For this review, take the finished solid that the model builds, in its own axes (mm). A direction names the side the tool comes from. Give positions to 0.01 mm unless a question says otherwise; leave off trailing zeros. Write each loop counter-clockwise with the first axis right and the second up, starting at its lowest first coordinate (ties: lowest second). Pieces come first, ordered by that corner, then holes. Notation, with made-up numbers: M 84.5,47.5 L 112.5,47.5 A25 ccw 112.5,82.5 Z; hole C 42.25,80 d10. An arc over 180 degrees is marked long. Use one line per item in the form item = value. Start each with the question number.
Q1. Consider section C-C on y = 25.5. Write out the cut boundary in (x, z), and give its area (3 significant figures).
Q2. Clearance check with flat-ended pins moving along their axes: pin 1 Ø24.5 at (x, y) = (-18.5, 43.5) entering from -Z; pin 2 Ø5 at (y, z) = (88.5, 21.5) entering from +X; pin 3 Ø6 at (x, z) = (102.5, -33.5) entering from +Y. State where each tip first meets the part, or that it passes through.
Q3. Tool access review of faces 1 (the flat face through (-2, 42, -90)), 2 (the cylindrical face through (-65.814, 98.409, -20.726)), 3 (the flat face through (-85, 87, -1)): name each direction out of +Z, -Z, +X, -X, +Y, -Y from which nothing blocks a thin tool from reaching the whole face with its end or side.
Q4. For probe 1 along X at (y, z) = (55, 80.5); probe 2 along Z at (x, y) = (-52, 57); probe 3 along Y at (x, z) = (-48.5, -60.5), list the stretches that pass through material, from the lowest coordinate up. Write a range as [from, to].
Q5. Consider section B-B on z = 0. Write out the cut boundary in (x, y), and give its area (3 significant figures).
Q6. Consider section A-A on x = 0. Write out the cut boundary in (y, z).
Q7. Consider section D-D on x = -112.5. Write out the cut boundary in (y, z), and give its area (3 significant figures).
Autodesk Inventor part; units mm, degrees
ref_plane "YZ Plane" through (0, 0, 0) normal (1, 0, 0) x (0, 1, 0)
ref_plane "XZ Plane" through (0, 0, 0) normal (0, 1, 0) x (-1, 0, 0)
ref_plane "XY Plane" through (0, 0, 0) normal (0, 0, 1) x (1, 0, 0)
sketch "Sketch1" plane through (0, 0, 0) normal (0, 0, 1) x (1, 0, 0)
  line L0 (-142.5, 102) -> (142.5, 102) construction
  line L1 (142.5, 102) -> (142.5, 82) construction
  line L2 (142.5, 0) -> (-142.5, 0)
  line L3 (-142.5, 0) -> (-142.5, 82)
  line L4 (-142.5, 82) -> (142.5, 82)
  line L5 (142.5, 82) -> (142.5, 0)
  line L6 (80, 0) -> (142.5, 41)
  circle A0 centre (115.876, 55.376) radius 26.624
  line L7 (-142.5, 82) -> (-142.5, 102) construction
  line L8 (-80, 0) -> (-142.5, 41)
  circle A1 centre (-115.876, 55.376) radius 26.624
  point P0 (0, 0)
  point P1 (0, 0)
  point P2 (-130.4796, 33.1146)
  point P3 (130.4796, 33.1146)
  point P4 (115.876, 82)
  point P5 (-115.876, 82)
  dimension "d7" = 285
  dimension "d8" = 102
  dimension "d9" = 82
  dimension "d13" = 80
  dimension "d14" = 80
extrude "Extrusion1" add sketch "Sketch1" along normal mid plane 180 contours L2 L8 A1 L4 A0 L6 | A0 | A1
sketch "Sketch2" plane through (-115.876, 82, 90) normal (0, 1, 0) x (1, 0, 0)
  line L0 (30.876, -5) -> (200.876, -5)
  line L1 (200.876, -5) -> (200.876, 185)
  line L2 (200.876, 185) -> (30.876, 185)
  line L3 (30.876, 185) -> (30.876, -5)
  line L4 (30.876, -5) -> (200.876, 185) construction
  point P0 (115.876, 90)
  point P1 (115.876, 90)
  dimension "d17" = 190
  dimension "d18" = 170
extrude "Extrusion2" add sketch "Sketch2" along normal blind 10
sketch "Sketch3" plane through (0, 0, 0) normal (0, 1, 0) x (-1, 0, 0)
  circle A0 centre (0, 0) radius 69
  dimension "d21" = 138
extrude "Extrusion3" add sketch "Sketch3" along normal blind 105
properties part number "Roller platform"
Working result:
q1.outline = M -118.87,-90 L 118.87,-90 L 118.87,90 L -118.87,90 Z
q1.area = 42,800 mm²
q2.pin_1 = -90
q2.pin_2 = 85
q2.pin_3 = 82
q3.face_1 = -Z, +X, -X, -Y
q3.face_2 = +Y
q3.face_3 = +Z, -Z, -X, +Y
q4.probe_1 = [-142.5, 142.5]
q4.probe_2 = [-90, 90]
q4.probe_3 = [0, 92]
q5.outline = M -130.48,33.11 L -80,0 L 80,0 L 130.48,33.11 A26.62 ccw 115.88,82 L 85,82 L 85,92 L 69,92 L 69,105 L -69,105 L -69,92 L -85,92 L -85,82 L -115.88,82 A26.62 ccw Z
q5.area = 23,900 mm²
q6.outline = M 0,-90 L 82,-90 L 82,-95 L 92,-95 L 92,-69 L 105,-69 L 105,69 L 92,69 L 92,95 L 82,95 L 82,90 L 0,90 Z
q7.outline = M 21.32,-90 L 82,-90 L 82,90 L 21.32,90 Z
q7.area = 10,900 mm²
